Design review of the part built by this model. Coordinates are the model's own, in mm. A direction names the side the tool comes from. Coordinates: 2 decimals unless noted, no trailing zeros. Loops run counter-clockwise (first coordinate to the right, second up) from the corner with the lowest first, then second, coordinate; pieces in that order, holes last. Notation, with made-up numbers: (28.25, -22) - (83.25, -22) arc R27 ccw to (83.25, 11) - close; hole circle Ø7 at (80.5, 30.5). An arc over 180 degrees is marked (long way). Answer in a Markdown table with one row per item. Add a question column.
(1) For faces 1 (the face through (-11.3, 431.8, -0.1)), 2 (the face through (0, 213, -11.112)), list the 3-axis set-ups (+Z, -Z, +X, -X, +Y, -Y) from which the entire face can be reached by the end or side of a thin tool; tool diameter is ignored.
(2) To check wall thickness, follow L1, parallel to Y at x = 0, z = -11.7; L2, parallel to Y at x = -11.8, z = 0; L3, parallel to Z at x = 0.25, y = 297.5. State the ranges of each line that lie inside material, in increasing order. Write a range as [from, to].
(3) We need section A-A, the plane y = 326. Write out the cut boundary in (x, z).
(4) The part is to be moulded in two halves that separate along X. For faces 3 (the face through (-11.112, 213, 0)), 4 (the face through (-11.3, 0, -0.1)), 5 (the face through (-12.7, 213, 0)), say which applies: released by +X, released by -X, zero draft, split by the parting line, or undercut.
(5) Clearance check with flat-ended pins moving along their axes: pin 1 (6.5 mm diameter, centred on y = 215.9, z = 0, fed in from -X); pin 2 (4 mm diameter, centred on y = 190.5, z = 0, fed in from +X) (3 decimals). State where each tip first meets the part, or that it passes through.
from build123d import *

# Parameters (mm, degrees)
SKETCH1_W                  = 25.4
SKETCH1_H                  = 25.4
SKETCH1_W_2                = 22.225
SKETCH1_H_2                = 22.225
BOSS_EXTRUDE1_DEPTH        = 431.8
F_7_0_201_DIAMETER_HOLE1_D = 5.1054
F_7_0_201_DIAMETER_HOLE2_D = 5.1054


with BuildPart() as part:
    # Sketch1 → Boss-Extrude1 (new body)
    with BuildSketch(Plane(origin=(0, 0, 0), x_dir=(1, 0, 0), z_dir=(0, 1, 0))):
        Rectangle(SKETCH1_W, SKETCH1_H)
        Rectangle(SKETCH1_W_2, SKETCH1_H_2, mode=Mode.SUBTRACT)
    extrude(amount=BOSS_EXTRUDE1_DEPTH)

    # #7 (0.201) Diameter Hole1 (through all)
    with Locations(Plane.XY.offset(12.7)):
        with Locations((0, 12.7), (0, 38.1), (0, 368.3), (0, 393.7), (0, 419.1)):
            Hole(F_7_0_201_DIAMETER_HOLE1_D / 2)

    # #7 (0.201) Diameter Hole2 (through all)
    with Locations(Plane(origin=(12.7, 0, 0), x_dir=(0, 0, -1), z_dir=(1, 0, 0))):
        with Locations((0, 165.1), (0, 190.5), (0, 215.9), (0, 241.3), (0, 266.7)):
            Hole(F_7_0_201_DIAMETER_HOLE2_D / 2)


solid = part.part
Responses:
| question | item | result |
|---|---|---|
| 1 | face 1 | +Z, -Z, +X, -X, +Y |
| 1 | face 2 | +Y, -Y |
| 2 | L1 | y = [0, 10.15], [15.25, 35.55], [40.65, 365.75], [370.85, 391.15], [396.25, 416.55], [421.65, 431.8] |
| 2 | L2 | y = [0, 162.55], [167.65, 187.95], [193.05, 213.35], [218.45, 238.75], [243.85, 264.15], [269.25, 431.8] |
| 2 | L3 | z = [-12.7, -11.11], [11.11, 12.7] |
| 3 | outline | (-12.7, -12.7) - (12.7, -12.7) - (12.7, 12.7) - (-12.7, 12.7) - close; hole (-11.11, -11.11) - (11.11, -11.11) - (11.11, 11.11) - (-11.11, 11.11) - close |
| 4 | face 3 | undercut |
| 4 | face 4 | zero draft |
| 4 | face 5 | released by -X |
| 5 | pin 1 | stops at x = -12.7 |
| 5 | pin 2 | passes through |
